Verification items for the finished model (mm, model axes). Face numbers are marked on the shaded views. Coordinates: 2 decimals unless noted, no trailing zeros. Write each loop counter-clockwise with the first axis right and the second up, starting at its lowest first coordinate (ties: lowest second). Pieces come first, ordered by that corner, then holes. Notation, with made-up numbers: (84, -37) -> (96, -37) arc R15 cw to (96, -32) -> close; hole circle Ø9 at (50.5, 73). An arc over 180 degrees is marked (long way). Answer in a Markdown table with one row per item.
```python
from build123d import *

# Parameters (mm, degrees)
F0_R     = 23.564799
F1_DEPTH = 12.7
F2_R     = 5.731585
F2_R_2   = 6.023249
F2_R_3   = 5.610998
F2_R_4   = 5.425092
F2_R_5   = 4.934707
F2_R_6   = 5.195112
F2_R_7   = 5.370794
F3_DEPTH = 25.4


with BuildPart() as f1:
    # F0 (on Right) → F1 (new body)
    with BuildSketch(Plane.YZ):
        with Locations((-5.052262, 21.17021)):
            Circle(F0_R)
    extrude(amount=F1_DEPTH)

    # F2 (on face) → F3 (cut)
    with BuildSketch(Plane.YZ.offset(12.7)):
        with Locations((-14.112254, 33.503115)):
            Circle(F2_R)
        with Locations((0, 32.565415)):
            Circle(F2_R_2)
        with Locations((-16.925359, 20.375287)):
            Circle(F2_R_3)
        with Locations((-3.641246, 21.312989)):
            Circle(F2_R_4)
        with Locations((9.017731, 21.469273)):
            Circle(F2_R_5)
        with Locations((2.922666, 10.216848)):
            Circle(F2_R_6)
        with Locations((-10.048877, 8.810295)):
            Circle(F2_R_7)
    extrude(amount=-F3_DEPTH, mode=Mode.SUBTRACT)


solid = f1.part
```
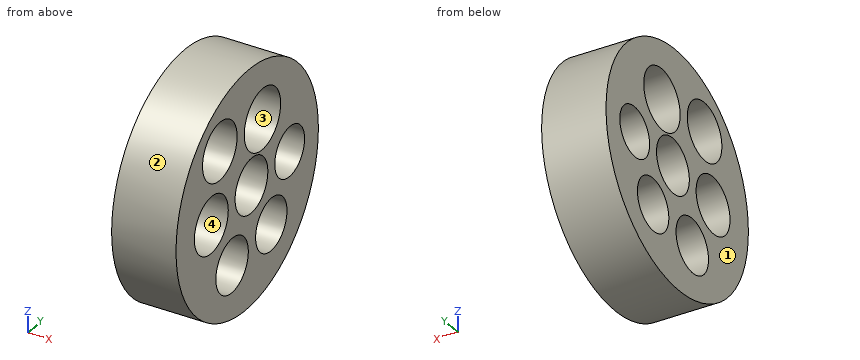
1. Sectioned sample at C-C, the plane y = 3.5. Record the cut outline in (x, z), and give its area (3 significant figures).
Findings below:
| item | result |
|---|---|
| outline | (0, -0.79) -> (12.7, -0.79) -> (12.7, 5.05) -> (0, 5.05) -> close; (0, 15.38) -> (12.7, 15.38) -> (12.7, 27.66) -> (0, 27.66) -> close; (0, 37.47) -> (12.7, 37.47) -> (12.7, 43.13) -> (0, 43.13) -> close |
| area | 302 mm² |
2. Material ranges on probe 1 along Y at (x, z) = (11, 19); probe 2 along Z at (x, y) = (11, -13.5); probe 3 along Y at (x, z) = (5, 5.5), recorded low to high. Write a range as from..to.
Findings below:
| item | result |
|---|---|
| probe 1 | y = -28.52..-22.37, -11.49..-8.55, 1.27..4.75, 13.29..18.41 |
| probe 2 | z = -0.83..4.7, 12.93..15.93, 24.82..27.8, 39.2..43.17 |
| probe 3 | y = -22.65..-14.28, -5.82..0.75, 5.1..12.55 |
3. Go/stop test with flat-tipped pins: pin 1 (1.5 mm diameter, centred on x = 2.5, y = -3.5, fed in from +Z); pin 2 (1.5 mm diameter, centred on x = 9.5, z = 4.5, fed in from -Y); pin 3 (1.5 mm diameter, centred on x = 9, z = 9, fed in from +Y). Record where each tip stops, or that it passes through.
Findings below:
| item | result |
|---|---|
| pin 1 | stops at z = 44.72 |
| pin 2 | stops at y = -22.43 |
| pin 3 | stops at y = 15.56 |
4. Sectioned sample at D-D, the plane x = 1.5. Record the cut outline in (y, z), and give its area (3 significant figures).
Findings below:
| item | result |
|---|---|
| outline | circle Ø47.13 at (-5.05, 21.17); hole circle Ø11.22 at (-16.93, 20.38); hole circle Ø11.46 at (-14.11, 33.5); hole circle Ø10.74 at (-10.05, 8.81); hole circle Ø10.85 at (-3.64, 21.31); hole circle Ø12.05 at (0, 32.57); hole circle Ø10.39 at (2.92, 10.22); hole circle Ø9.87 at (9.02, 21.47) |
| area | 1,080 mm² |
5. Sectioned sample at A-A, the plane z = 30. Record the cut outline in (x, y), and give its area (3 significant figures).
Findings below:
| item | result |
|---|---|
| outline | (0, -26.9) -> (12.7, -26.9) -> (12.7, -18.65) -> (0, -18.65) -> close; (0, -9.58) -> (12.7, -9.58) -> (12.7, -5.45) -> (0, -5.45) -> close; (0, 5.45) -> (12.7, 5.45) -> (12.7, 16.8) -> (0, 16.8) -> close |
| area | 301 mm² |
6. Release check for a two-part mould opening along Z. For the marked faces 1, 2, 3 and 4 record: released by +Z, released by -Z, zero draft, split by the parting line, or undercut.
Findings below:
| item | result |
|---|---|
| face 1 | zero draft |
| face 2 | split by the parting line |
| face 3 | undercut |
| face 4 | undercut |
7. Sectioned sample at B-B, the plane z = 23.5. Record the cut outline in (x, y), and give its area (3 significant figures).
Findings below:
| item | result |
|---|---|
| outline | (0, -28.5) -> (12.7, -28.5) -> (12.7, -21.59) -> (0, -21.59) -> close; (0, -12.26) -> (12.7, -12.26) -> (12.7, -8.61) -> (0, -8.61) -> close; (0, 1.32) -> (12.7, 1.32) -> (12.7, 4.52) -> (0, 4.52) -> close; (0, 13.52) -> (12.7, 13.52) -> (12.7, 18.4) -> (0, 18.4) -> close |
| area | 237 mm² |
